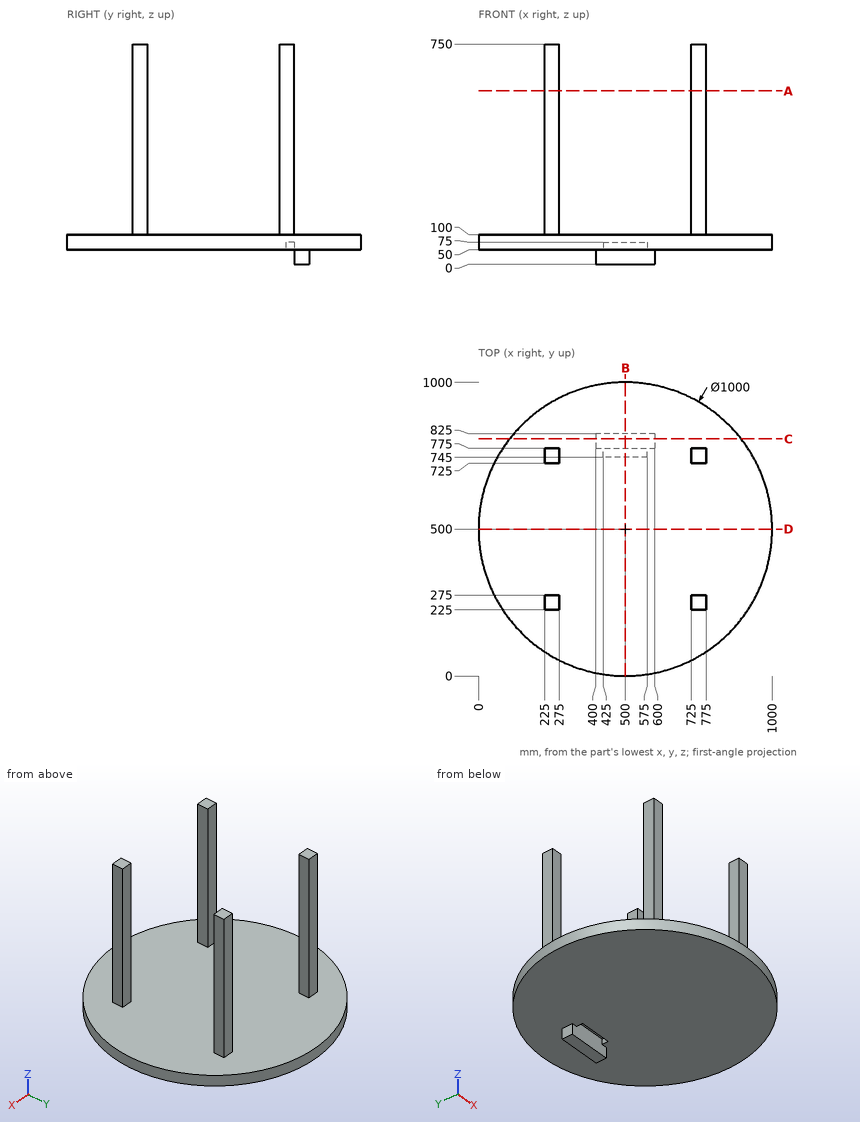
For this review, use the dimensioned drawing (mm, ordinates from the lowest corner) and the shaded views. Coordinates: 2 decimals unless noted, no trailing zeros. Loops run counter-clockwise (first coordinate to the right, second up) from the corner with the lowest first, then second, coordinate; pieces in that order, holes last.
1. Add section D-D, the plane y = 500. Give the boundary of the cut face in (x, z), then the cut area to 3 significant figures.
2. Add section A-A, the plane z = 590. Give the boundary of the cut face in (x, y).
3. For line 1 (Y direction, x = 732.5, z = 268.5); line 2 (Z direction, x = 240, y = 514), list the stretches that pass through material, from the lowest coordinate up.
4. Insertion check: P1, Ø15, axis at y = 762.5, z = 471.5, coming from the -X side; P2, Ø7.5, axis at y = 765, z = 60, coming from the +X side; P3, Ø25, axis at x = 259.5, z = 425.5, coming from the +Y side. Each pin has a flat end and moves straight along its axis. Give the tip position at first contact, or say it passes through.
5. Add section B-B, the plane x = 500. Give the boundary of the cut face in (y, z).
6. Add section C-C, the plane y = 807. Give the boundary of the cut face in (x, z), then the cut area to 3 significant figures.
Result:
1. outline: (0, 50) - (1000, 50) - (1000, 100) - (0, 100) - close
1. area: 50,000 mm2
2. outline: (225, 225) - (275, 225) - (275, 275) - (225, 275) - close; (225, 725) - (275, 725) - (275, 775) - (225, 775) - close; (725, 225) - (775, 225) - (775, 275) - (725, 275) - close; (725, 725) - (775, 725) - (775, 775) - (725, 775) - close
3. line 1: y = 225 to 275, 725 to 775
3. line 2: z = 50 to 100
4. P1: stops at x = 225
4. P2: stops at x = 926.32
4. P3: stops at y = 775
5. outline: (0, 50) - (745, 50) - (745, 75) - (775, 75) - (775, 0) - (825, 0) - (825, 50) - (1000, 50) - (1000, 100) - (0, 100) - close
6. outline: (105.35, 50) - (400, 50) - (400, 0) - (600, 0) - (600, 50) - (894.65, 50) - (894.65, 100) - (105.35, 100) - close
6. area: 49,500 mm2
